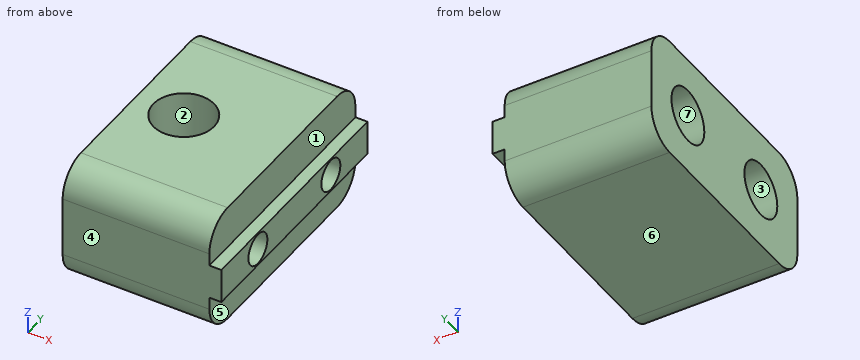
```python
from build123d import *

# Parameters (mm, degrees)
F0_W     = 24.392
F0_H     = 40
F1_DEPTH = 20
F2_R     = 5.05
F3_DEPTH = 10
F4_W     = 40
F4_H     = 5.8
F5_DEPTH = 2
F6_R     = 2.6
F7_DEPTH = 26.393
F8_R     = 4.5
F9_DEPTH = 20.4
F10_R    = 5


with BuildPart() as f1:
    # F0 (on Top) → F1 (new body)
    with BuildSketch(Plane.XY):
        with Locations((4.196, 0)):
            Rectangle(F0_W, F0_H)
    extrude(amount=F1_DEPTH)

    # F2 (on face) → F3 (cut)
    with BuildSketch(Plane.XY.offset(20)):
        Circle(F2_R)
    extrude(amount=-F3_DEPTH, mode=Mode.SUBTRACT)

    # F4 (on face) → F5 (join)
    with BuildSketch(Plane.YZ.offset(16.392)):
        with Locations((0, 10)):
            Rectangle(F4_W, F4_H)
    extrude(amount=F5_DEPTH)

    # F6 (on face) → F7 (cut, through all)
    with BuildSketch(Plane(origin=(-8, 0, 0), x_dir=(0, -1, 0), z_dir=(-1, 0, 0))):
        with Locations((-10, 10)):
            Circle(F6_R)
        with Locations((10, 10)):
            Circle(F6_R)
    extrude(amount=-F7_DEPTH, mode=Mode.SUBTRACT)

    # F8 (on face) → F9 (cut)
    with BuildSketch(Plane(origin=(-8, 0, 0), x_dir=(0, -1, 0), z_dir=(-1, 0, 0))):
        with Locations((-10, 10)):
            Circle(F8_R)
        with Locations((10, 10)):
            Circle(F8_R)
    extrude(amount=-F9_DEPTH, mode=Mode.SUBTRACT)

    # F10
    f10_edges = [f1.edges().sort_by_distance(p)[0] for p in [
        (4.196, -20, 20),
        (4.196, 20, 20),
        (4.196, -20, 0),
        (4.196, 20, 0),
    ]]
    fillet(f10_edges, radius=F10_R)


solid = f1.part
```
For this review, take the finished solid that the model builds, in its own axes (mm). Face numbers are marked on the shaded views. A direction names the side the tool comes from. Round coordinates to 2 decimals unless told otherwise and drop trailing zeros. Order: outer loops, then holes, each group sorted by start corner. A loop starts at its lowest first (then second) coordinate and runs counter-clockwise, first axis right, second up. Notation, with made-up numbers: (62, 30) -> (97, 30) arc R24 ccw to (97, 43) -> close; hole circle Ø4 at (73.5, 60.25). An arc over 180 degrees is marked (long way). Use a Markdown table: item, result.
Item 1: For pin 1 (4.5 mm diameter, centred on y = -10, z = 10, fed in from -X); pin 2 (8 mm diameter, centred on y = 3, z = 3.5, fed in from +X); pin 3 (0.6 mm diameter, centred on x = 17.5, y = -7.5, fed in from -Z); pin 4 (4.5 mm diameter, centred on y = 11, z = 11, fed in from -X), all flat-tipped, find the tip position at first contact; note any pin that passes through.
Resolved:
| item | result |
|---|---|
| pin 1 | passes through |
| pin 2 | stops at x = 18.39 |
| pin 3 | stops at z = 7.1 |
| pin 4 | stops at x = 12.4 |
Item 2: Take a section at A-A (y = 10). State the section outline as (x, z) points, plus the area to 3 significant figures.
Resolved:
| item | result |
|---|---|
| outline | (-8, 0) -> (16.39, 0) -> (16.39, 7.1) -> (18.39, 7.1) -> (18.39, 7.4) -> (12.4, 7.4) -> (12.4, 5.5) -> (-8, 5.5) -> close; (-8, 14.5) -> (12.4, 14.5) -> (12.4, 12.6) -> (18.39, 12.6) -> (18.39, 12.9) -> (16.39, 12.9) -> (16.39, 20) -> (-8, 20) -> close |
| area | 285 mm² |
Item 3: Take a section at D-D (y = 0). State the section outline as (x, z) points, plus the area to 3 significant figures.
Resolved:
| item | result |
|---|---|
| outline | (-8, 0) -> (16.39, 0) -> (16.39, 7.1) -> (18.39, 7.1) -> (18.39, 12.9) -> (16.39, 12.9) -> (16.39, 20) -> (5.05, 20) -> (5.05, 10) -> (-5.05, 10) -> (-5.05, 20) -> (-8, 20) -> close |
| area | 398 mm² |
Item 4: Take a section at C-C (z = 18). State the section outline as (x, y) points.
Resolved:
| item | result |
|---|---|
| outline | (-8, -19) -> (16.39, -19) -> (16.39, 19) -> (-8, 19) -> close; hole circle Ø10.1 at (0, 0) |
Item 5: For line 1 along Y through (x, z) = (-4.75, 7.75); line 2 along Z through (x, y) = (16.45, -10); line 3 along Y through (x, z) = (4, 13), list the stretches that pass through material, from the lowest coordinate up. Write a range as [from, to].
Resolved:
| item | result |
|---|---|
| line 1 | y = [-20, -13.9], [-6.1, 6.1], [13.9, 20] |
| line 2 | z = [7.1, 7.4], [12.6, 12.9] |
| line 3 | y = [-20, -13.35], [-6.65, -3.08], [3.08, 6.65], [13.35, 20] |
Item 6: Take a section at B-B (x = -0.75). State the section outline as (y, z) points.
Resolved:
| item | result |
|---|---|
| outline | (-20, 5) arc R5 ccw to (-15, 0) -> (15, 0) arc R5 ccw to (20, 5) -> (20, 15) arc R5 ccw to (15, 20) -> (4.99, 20) -> (4.99, 10) -> (-4.99, 10) -> (-4.99, 20) -> (-15, 20) arc R5 ccw to (-20, 15) -> close; hole circle Ø9 at (-10, 10); hole circle Ø9 at (10, 10) |
Item 7: Draft analysis for pull direction Z (two halves, no side actions). For the marked faces 5, 6 and 7, state which applies: +Z half, -Z half, draft (parallel to the pull), parting line (faces both ways), or undercut.
Resolved:
| item | result |
|---|---|
| face 5 | draft |
| face 6 | -Z half |
| face 7 | undercut |
Item 8: Machinability: for the marked faces 1, 2, 3 and 4, which of the approach directions +Z, -Z, +X, -X, +Y, -Y give a long, thin tool a straight path to every point of the face, cutting with its end or side? Answer none if there is none.
Resolved:
| item | result |
|---|---|
| face 1 | +Z, +X, +Y, -Y |
| face 2 | +Z |
| face 3 | -X |
| face 4 | +Z, -Z, +X, -X, -Y |
